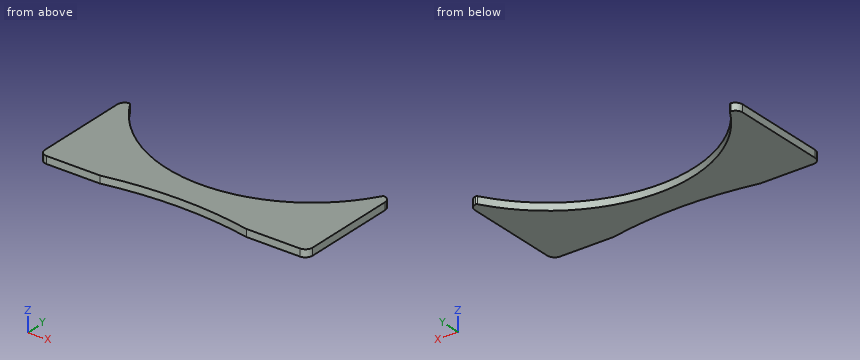
Autodesk Inventor part; units mm, degrees
ref_plane "YZ Plane" through (0, 0, 0) normal (1, 0, 0) x (0, 1, 0)
ref_plane "XZ Plane" through (0, 0, 0) normal (0, 1, 0) x (-1, 0, 0)
ref_plane "XY Plane" through (0, 0, 0) normal (0, 0, 1) x (1, 0, 0)
sketch "Skizze1" plane through (0, 0, 0) normal (0, 0, 1) x (1, 0, 0)
  circle A0 centre (0, 0) radius 100 construction
  arc A1 (-86.2926, -50.5331) -> (86.2926, -50.5331) centre (0, 0) ccw
  line L0 (-86.6025, -50) -> (0, 0) construction
  line L1 (0, 0) -> (86.6025, -50) construction
  line L2 (0, -467) -> (0, 194.5) construction
  line L3 (-86.6025, -125) -> (86.6025, -125)
  line L4 (-86.6025, -50) -> (-86.6025, -50)
  line L5 (-91.6025, -55) -> (-91.6025, -120)
  line L6 (86.6025, -50) -> (86.6025, -50)
  line L7 (91.6025, -55) -> (91.6025, -120)
  arc A2 (-87.2937, -50.048) -> (-91.6025, -55) centre (-86.6025, -55) ccw
  arc A3 (91.6025, -55) -> (87.2937, -50.048) centre (86.6025, -55) ccw
  arc A4 (-86.2926, -50.5331) -> (-87.2937, -50.048) centre (-87.1555, -51.0384) ccw
  arc A5 (87.2937, -50.048) -> (86.2926, -50.5331) centre (87.1555, -51.0384) ccw
  arc A6 (-91.6025, -120) -> (-86.6025, -125) centre (-86.6025, -120) ccw
  arc A7 (86.6025, -125) -> (91.6025, -120) centre (86.6025, -120) ccw
  arc A8 (50, -125) -> (-50, -125) centre (0, -372.5) ccw
  point P0 (0, -100)
  point P1 (-91.6025, -50)
  point P2 (0, -125)
  point P3 (0, -120)
  dimension "d0" = 200
  dimension "d1" = 60
  dimension "d2" = 5
  dimension "d3" = 25
  dimension "d4" = 5
  dimension "d5" = 1
  dimension "d6" = 5
  dimension "d7" = 50
  dimension "d8" = 50
  dimension "d9" = 5
extrude "Extrusion1" add sketch "Skizze1" along normal blind 5 contours A1 A5 A3 L7 A7 L3 A8 A6 L5 A2 A4
properties part number "Montage_Fuss"
For this review, take the finished solid that the model builds, in its own axes (mm). Round coordinates to 2 decimals unless told otherwise and drop trailing zeros. Order: outer loops, then holes, each group sorted by start corner. A loop starts at its lowest first (then second) coordinate and runs counter-clockwise, first axis right, second up. Notation, with made-up numbers: (65, -25) -> (117, -25) arc R6 cw to (117, -21) -> close; hole circle Ø4 at (53, 11). An arc over 180 degrees is marked (long way). Use a Markdown table: item, result.
Item 1: Take a section at B-B (y = -57). State the section outline as (x, z) points.
Resolved:
| item | result |
|---|---|
| outline | (-91.6, 0) -> (-82.16, 0) -> (-82.16, 5) -> (-91.6, 5) -> close; (82.16, 0) -> (91.6, 0) -> (91.6, 5) -> (82.16, 5) -> close |
Item 2: Take a section at D-D (x = -30). State the section outline as (y, z) points.
Resolved:
| item | result |
|---|---|
| outline | (-121.79, 0) -> (-95.39, 0) -> (-95.39, 5) -> (-121.79, 5) -> close |
Item 3: Take a section at C-C (y = -78). State the section outline as (x, z) points.
Resolved:
| item | result |
|---|---|
| outline | (-91.6, 0) -> (-62.58, 0) -> (-62.58, 5) -> (-91.6, 5) -> close; (62.58, 0) -> (91.6, 0) -> (91.6, 5) -> (62.58, 5) -> close |
Item 4: For pin 1 (5 mm diameter, centred on x = -48.5, y = -97.5, fed in from -Z), flat-tipped, find the tip position at first contact; note if it passes through.
Resolved:
| item | result |
|---|---|
| pin 1 | stops at z = 0 |
Item 5: For line 1 along Y through (x, z) = (50, 3.45); line 2 along X through (y, z) = (-83.5, 2.1); line 3 along Y through (x, z) = (-1, 2), list the stretches that pass through material, from the lowest coordinate up. Write a range as [from, to].
Resolved:
| item | result |
|---|---|
| line 1 | y = [-125, -86.6] |
| line 2 | x = [-91.6, -55.03], [55.03, 91.6] |
| line 3 | y = [-120, -100] |
Item 6: Take a section at A-A (z = 1.9). State the section outline as (x, y) points.
Resolved:
| item | result |
|---|---|
| outline | (-91.6, -120) arc R5 ccw to (-86.6, -125) -> (-50, -125) arc R252.5 cw to (50, -125) -> (86.6, -125) arc R5 ccw to (91.6, -120) -> (91.6, -55) arc R5 ccw to (87.29, -50.05) arc R1 ccw to (86.29, -50.53) arc R100 cw to (-86.29, -50.53) arc R1 ccw to (-87.29, -50.05) arc R5 ccw to (-91.6, -55) -> close |
